Study the drawing (mm; zero at the part's minimum x, y, z) and answer. A direction names the side the tool comes from. Give positions to 0.01 mm unless a question says otherwise; leave off trailing zeros. Write each loop counter-clockwise with the first axis right and the second up, starting at its lowest first coordinate (ties: lowest second). Pieces come first, ordered by that corner, then holes. Notation, with made-up numbers: M 59,12.5 L 117,12.5 A19 ccw 117,25.5 Z; hole C 41.5,76.5 d10. An arc over 180 degrees is marked long. Use a Markdown table: item, result. Add a question column.
Item 1: Given P1, Ø4, axis at x = 180, z = 62.5, coming from the +Y side; P2, Ø8, axis at x = 45, y = 52.5, coming from the -Z side; P3, Ø2, axis at x = 254, y = 58.5, coming from the -Z side; P4, Ø5, axis at x = 123.5, y = 46, coming from the -Z side, each flat-ended and moving along its own axis, determine where each tip first touches the part or whether it passes through.
Item 2: A cutting plane is placed at B-B on z = 84. Determine the outline of the cut face in (x, y), then the cut area to 3 significant figures.
Item 3: The mould has two halves that part along X. Classify the marked faces 4, 5 and 6: pulls with the +X half, pulls with the -X half, needs draft (parallel to the pull), parting line crosses it, or undercut.
Item 4: For the marked faces 1, 2 and 3, determine the directions among +Z, -Z, +X, -X, +Y, -Y from which every point of the face is accessible in a straight line to the end or side of a thin tool.
Item 5: A cutting plane is placed at D-D on z = 31.5. Determine the outline of the cut face in (x, y).
Item 6: A cutting plane is placed at A-A on y = 9.5. Determine the outline of the cut face in (x, z) (1 decimal), then the cut area to 3 significant figures.
Item 7: A cutting plane is placed at C-C on x = 244.5. Determine the outline of the cut face in (y, z) (1 decimal).
Item 8: Consider probe 1 along X at (y, z) = (35, 90); probe 2 along X at (y, z) = (32, 78) (1 decimal); probe 3 along Y at (x, z) = (107, 42). Determine where each line is inside the solid, lowest interval first. Write a range as [from, to].
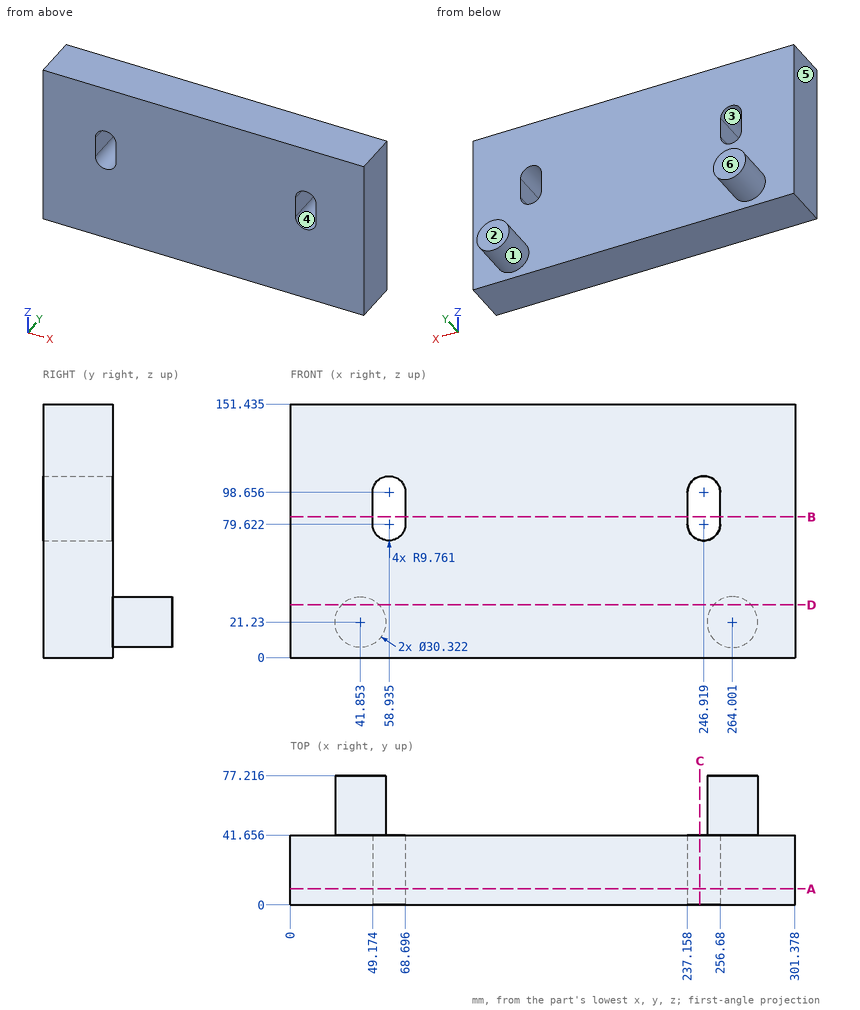
Filled in:
| question | item | result |
|---|---|---|
| 1 | P1 | y = 41.66 |
| 1 | P2 | z = 6.07 |
| 1 | P3 | z = 9.03 |
| 1 | P4 | through |
| 2 | outline | M 0,0 L 49.17,0 L 49.17,41.66 L 0,41.66 Z; M 68.7,0 L 237.16,0 L 237.16,41.66 L 68.7,41.66 Z; M 256.68,0 L 301.38,0 L 301.38,41.66 L 256.68,41.66 Z |
| 2 | area | 10,900 mm² |
| 3 | face 4 | undercut |
| 3 | face 5 | pulls with the -X half |
| 3 | face 6 | needs draft |
| 4 | face 1 | +Y |
| 4 | face 2 | +Z, -Z, +X, -X, +Y |
| 4 | face 3 | +Y, -Y |
| 5 | outline | M 0,0 L 301.38,0 L 301.38,41.66 L 275.15,41.66 L 275.15,77.22 L 252.85,77.22 L 252.85,41.66 L 53.01,41.66 L 53.01,77.22 L 30.7,77.22 L 30.7,41.66 L 0,41.66 Z |
| 6 | outline | M 0,0 L 301.4,0 L 301.4,151.4 L 0,151.4 Z; hole M 49.2,79.6 A9.8 ccw 68.7,79.6 L 68.7,98.7 A9.8 ccw 49.2,98.7 Z; hole M 237.2,79.6 A9.8 ccw 256.7,79.6 L 256.7,98.7 A9.8 ccw 237.2,98.7 Z |
| 6 | area | 44,300 mm² |
| 7 | outline | M 0,0 L 41.7,0 L 41.7,70.2 L 0,70.2 Z; M 0,108.1 L 41.7,108.1 L 41.7,151.4 L 0,151.4 Z |
| 8 | probe 1 | [0, 49.17], [68.7, 237.16], [256.68, 301.38] |
| 8 | probe 2 | [0, 49.3], [68.6, 237.3], [256.5, 301.4] |
| 8 | probe 3 | [0, 41.66] |
